Autodesk Inventor part; units mm, degrees
ref_plane "YZ Plane" through (0, 0, 0) normal (1, 0, 0) x (0, 1, 0)
ref_plane "XZ Plane" through (0, 0, 0) normal (0, 1, 0) x (-1, 0, 0)
sketch "스케치1" plane through (0, 0, 0) normal (0, 0, 1) x (1, 0, 0)
  line L0 (0, 0) -> (0, -26)
  line L1 (0, 0) -> (26, 0) construction
  arc A0 (-9.5556, -30.833) -> (0, -26) centre (-6, -26) ccw
  line L2 (0, 0) -> (-15.2463, 17)
  arc A1 (-15.2463, 17) -> (-9.5556, -30.833) centre (10, -4.2514) ccw
  circle A2 centre (-6, -26) radius 3
  dimension "d1" = 26
  dimension "d3" = 26
  dimension "d5" = 43
  dimension "d6" = 23
  dimension "d7" = 33
  dimension "d8" = 6
  dimension "d9" = 6
extrude "돌출1" add sketch "스케치1" along normal mid plane 16
ref_plane "작업 평면1" through (0, 0, 0) normal (0, 0, -1) x (-1, 0, 0)
sketch "스케치2" plane through (0, 0, 0) normal (0, 0, -1) x (-1, 0, 0)
  arc A0 (9.5556, -30.833) -> (15.2463, 17) centre (-10, -4.2514) ccw
  line L0 (22.8853, -7) -> (17.8648, -7)
  line L1 (0, 0) -> (0, -26)
  circle A1 centre (6, -26) radius 3
  arc A2 (17.8648, -7) -> (11.869, 13.2342) centre (-10, -4.2514) ccw
  line L2 (15.2463, 17) -> (0, 0)
  arc A3 (0, -26) -> (9.5556, -30.833) centre (6, -26) ccw
  dimension "d14" = 19
extrude "돌출2" cut sketch "스케치2" along normal mid plane 8 contours A3 L1 L2 A2 L0 A0
sketch "스케치6" plane through (0, 0, 8) normal (0, 0, 1) x (1, 0, 0)
  line L0 (-18.2733, -4.3259) -> (-3.2652, -4.3259) construction
  line L1 (-3.2652, -4.3259) -> (-3.2652, -14.7392) construction
  line L2 (-3.2652, -14.7392) -> (-18.2733, -14.7392) construction
  line L3 (-18.2733, -14.7392) -> (-18.2733, -4.3259) construction
  spline S0 degree 2 poles (-11.4824, -11.3519) (-11.4824, -12.0731) (-11.9443, -13.3049) (-12.3657, -13.7587) knots 0 0 0 1 2 2 2
  spline S1 degree 2 poles (-12.3657, -13.7587) (-12.7871, -14.2125) (-14.0432, -14.7392) (-14.8212, -14.7392) knots 0 0 0 1 2 2 2
  spline S2 degree 2 poles (-14.8212, -14.7392) (-15.5343, -14.7392) (-16.9281, -14.4232) (-17.4387, -14.172) knots 0 0 0 1 2 2 2
  line L4 (-17.4387, -14.172) -> (-17.4387, -12.7538)
  line L5 (-17.4387, -12.7538) -> (-17.3414, -12.7538)
  spline S3 degree 2 poles (-17.3414, -12.7538) (-17.1874, -12.8673) (-16.6121, -13.159) (-16.2636, -13.2887) knots 0 0 0 1 2 2 2
  spline S4 degree 2 poles (-16.2636, -13.2887) (-15.8665, -13.4264) (-15.2101, -13.5804) (-14.7968, -13.5804) knots 0 0 0 1 2 2 2
  spline S5 degree 2 poles (-14.7968, -13.5804) (-14.3917, -13.5804) (-13.6299, -13.2887) (-13.3544, -12.9726) knots 0 0 0 1 2 2 2
  spline S6 degree 2 poles (-13.3544, -12.9726) (-13.1032, -12.6728) (-12.8439, -11.8786) (-12.8439, -11.3438) knots 0 0 0 1 2 2 2
  spline S7 degree 2 poles (-12.8439, -11.3438) (-12.8439, -10.8089) (-13.1356, -10.1282) (-13.4111, -9.9013) knots 0 0 0 1 2 2 2
  spline S8 degree 2 poles (-13.4111, -9.9013) (-13.6947, -9.6501) (-14.5375, -9.4394) (-15.0481, -9.4394) knots 0 0 0 1 2 2 2
  spline S9 degree 2 poles (-15.0481, -9.4394) (-15.5991, -9.4394) (-16.6931, -9.6096) (-17.0254, -9.6825) knots 0 0 0 1 2 2 2
  line L6 (-17.0254, -9.6825) -> (-17.0254, -4.5285)
  line L7 (-17.0254, -4.5285) -> (-11.5392, -4.5285)
  line L8 (-11.5392, -4.5285) -> (-11.5392, -5.7036)
  line L9 (-11.5392, -5.7036) -> (-15.7369, -5.7036)
  line L10 (-15.7369, -5.7036) -> (-15.7369, -8.3697)
  spline S10 degree 2 poles (-15.7369, -8.3697) (-15.4938, -8.3373) (-15.0238, -8.313) (-14.8293, -8.313) knots 0 0 0 1 2 2 2
  spline S11 degree 2 poles (-14.8293, -8.313) (-14.0594, -8.313) (-12.9978, -8.5642) (-12.5116, -8.937) knots 0 0 0 1 2 2 2
  spline S12 degree 2 poles (-12.5116, -8.937) (-12.0173, -9.3097) (-11.4824, -10.4442) (-11.4824, -11.3519) knots 0 0 0 1 2 2 2
  spline S13 degree 2 poles (-3.8163, -9.5285) (-3.8163, -12.219) (-5.3803, -14.7392) (-7.0092, -14.7392) knots 0 0 0 1 2 2 2
  spline S14 degree 2 poles (-7.0092, -14.7392) (-8.6623, -14.7392) (-10.2101, -12.1703) (-10.2101, -9.5366) knots 0 0 0 1 2 2 2
  spline S15 degree 2 poles (-10.2101, -9.5366) (-10.2101, -6.83) (-8.6461, -4.3259) (-7.0092, -4.3259) knots 0 0 0 1 2 2 2
  spline S16 degree 2 poles (-7.0092, -4.3259) (-5.3641, -4.3259) (-3.8163, -6.9191) (-3.8163, -9.5285) knots 0 0 0 1 2 2 2
  spline S17 degree 2 poles (-5.5343, -12.5755) (-5.3398, -12.0812) (-5.1777, -10.5577) (-5.1777, -9.5285) knots 0 0 0 1 2 2 2
  spline S18 degree 2 poles (-5.1777, -9.5285) (-5.1777, -8.4994) (-5.3398, -6.984) (-5.5424, -6.4734) knots 0 0 0 1 2 2 2
  spline S19 degree 2 poles (-5.5424, -6.4734) (-5.745, -5.9629) (-6.45, -5.4361) (-7.0092, -5.4361) knots 0 0 0 1 2 2 2
  spline S20 degree 2 poles (-7.0092, -5.4361) (-7.5683, -5.4361) (-8.2896, -5.9629) (-8.5003, -6.4896) knots 0 0 0 1 2 2 2
  spline S21 degree 2 poles (-8.5003, -6.4896) (-8.7028, -7.0002) (-8.8487, -8.5561) (-8.8487, -9.5366) knots 0 0 0 1 2 2 2
  spline S22 degree 2 poles (-8.8487, -9.5366) (-8.8487, -10.5901) (-8.7191, -12.0002) (-8.5084, -12.5512) knots 0 0 0 1 2 2 2
  spline S23 degree 2 poles (-8.5084, -12.5512) (-8.3139, -13.0699) (-7.5926, -13.629) (-7.0092, -13.629) knots 0 0 0 1 2 2 2
  spline S24 degree 2 poles (-7.0092, -13.629) (-6.4581, -13.629) (-5.7369, -13.1023) (-5.5343, -12.5755) knots 0 0 0 1 2 2 2
  point P0 (0, 0)
extrude "돌출3" cut sketch "스케치6" against normal blind 1
properties part number "05-1"
Geometry check sheet. Reference: the model listing, model coordinates, mm. A direction names the side the tool comes from. Round coordinates to 2 decimals unless told otherwise and drop trailing zeros. Order: outer loops, then holes, each group sorted by start corner. A loop starts at its lowest first (then second) coordinate and runs counter-clockwise, first axis right, second up. Notation, with made-up numbers: M -23.75,14.5 L -8.75,14.5 A23 cw -8.75,34.5 Z; hole C 58.25,73 d7. An arc over 180 degrees is marked long. Answer in a Markdown table with one row per item.
(1) Sectioned sample at B-B, the plane z = 6. Record the cut outline in (x, y), and give its area (3 significant figures).
Responses:
| item | result |
|---|---|
| outline | M -15.25,17 A33 ccw -9.56,-30.83 A6 ccw 0,-26 L 0,0 Z; hole C -6,-26 d6 |
| area | 785 mm² |
(2) Sectioned sample at D-D, the plane y = 3. Record the cut outline in (x, z).
Responses:
| item | result |
|---|---|
| outline | M -22.19,-8 L -2.69,-8 L -2.69,-4 L -17.04,-4 L -17.04,4 L -2.69,4 L -2.69,8 L -22.19,8 Z |
(3) Tool access check on faces 4 (the face through (-9, -9, -4)), 5 (the face through (-13, -10, 7)), 6 (the face through (-20, -7, 0)). Record the directions out of +Z, -Z, +X, -X, +Y, -Y that give a thin tool (end or side, any length) a straight path to the whole face; none if there is none.
Responses:
| item | result |
|---|---|
| face 4 | +X, -Y |
| face 5 | +Z |
| face 6 | +X, -X, -Y |
(4) Sectioned sample at A-A, the plane y = -16.5. Record the cut outline in (x, z), and give its area (3 significant figures).
Responses:
| item | result |
|---|---|
| outline | M -20.64,-8 L 0,-8 L 0,-4 L -20.64,-4 Z; M -20.64,4 L 0,4 L 0,8 L -20.64,8 Z |
| area | 165 mm² |
(5) Go/stop test with flat-tipped pins: P1, Ø1.5, axis at y = 12, z = -4, coming from the -X side; P2, Ø6, axis at x = -11.5, z = 2, coming from the +Y side; P3, Ø1.1, axis at x = -13, z = 7.5, coming from the +Y side; P4, Ø6, axis at x = -19.5, y = -27, coming from the +Z side. Record where each tip stops, or that it passes through.
Responses:
| item | result |
|---|---|
| P1 | stops at x = -19.13 |
| P2 | stops at y = 16.17 |
| P3 | stops at y = 15.11 |
| P4 | passes through |
(6) Scan lines: probe 1 along X at (y, z) = (-26, -6.65); probe 2 along Z at (x, y) = (-10.5, 8); probe 3 along Z at (x, y) = (-16.5, -8). Record each from-to range of solid material in increasing order. Write a range as from..to.
Responses:
| item | result |
|---|---|
| probe 1 | x = -14.82..-9, -3..0 |
| probe 2 | z = -8..-4, 4..8 |
| probe 3 | z = -8..-4, 4..7 |
(7) Sectioned sample at C-C, the plane x = -21.5. Record the cut outline in (y, z), and give its area (3 significant figures).
Responses:
| item | result |
|---|---|
| outline | M -14.09,-8 L 5.58,-8 L 5.58,8 L -14.09,8 L -14.09,4 L -7,4 L -7,-4 L -14.09,-4 Z |
| area | 258 mm² |
(8) Draft check along Y on faces 1 (the face through (-3.21, -31.31, 5.97)), 2 (the face through (-14.3, -4.528, 7.5)), 3 (the face through (-12, -7, 8)). Enter one of: released by +Y, released by -Y, zero draft, split by the parting line, or undercut.
Responses:
| item | result |
|---|---|
| face 1 | released by -Y |
| face 2 | undercut |
| face 3 | zero draft |
